from build123d import *

# Parameters (mm, degrees)
SKETCH2_R           = 6
BOSS_EXTRUDE1_DEPTH = 20


with BuildPart() as part:
    # Sketch2 → Boss-Extrude1 (new body)
    with BuildSketch(Plane(origin=(0, 0, 0), x_dir=(1, 0, 0), z_dir=(0, 1, 0))):
        with BuildLine():
            ThreePointArc((150, 0), (105, 77.942286341), (15, 77.942286341))
            ThreePointArc((15, 77.942286341), (7.764571353, 74.945273665), (0, 73.923048454))
            ThreePointArc((0, 73.923048454), (-7.764571353, 74.945273665), (-15, 77.942286341))
            ThreePointArc((-15, 77.942286341), (-150, 0), (-15, -77.942286341))
            ThreePointArc((-15, -77.942286341), (-7.764571353, -74.945273665), (0, -73.923048454))
            ThreePointArc((0, -73.923048454), (7.764571353, -74.945273665), (15, -77.942286341))
            ThreePointArc((15, -77.942286341), (105, -77.942286341), (150, 0))
        make_face()
        with Locations((60, 0)):
            Circle(SKETCH2_R, mode=Mode.SUBTRACT)
        with Locations((-60, 0)):
            Circle(SKETCH2_R, mode=Mode.SUBTRACT)
        with BuildLine():
            Line((5, 60.048226517), (5, 20))
            ThreePointArc((5, 20), (6.464466094, 16.464466094), (10, 15))
            Line((10, 15), (65.857864376, 15))
            ThreePointArc((65.857864376, 15), (67.771281538, 15.380602337), (69.393398282, 16.464466094))
            Line((69.393398282, 16.464466094), (109.023956198, 56.09502401))
            ThreePointArc((109.023956198, 56.09502401), (110.47724887, 59.964637812), (108.520983778, 63.605928444))
            ThreePointArc((108.520983778, 63.605928444), (65.119211843, 79.836042425), (20, 69.282032303))
            ThreePointArc((20, 69.282032303), (14.607936726, 66.68586026), (8.888888889, 64.923206732))
            ThreePointArc((8.888888889, 64.923206732), (6.0913202, 63.166274339), (5, 60.048226517))
        make_face(mode=Mode.SUBTRACT)
        with BuildLine():
            Line((134.330343737, 5), (73.036753237, 5))
            ThreePointArc((73.036753237, 5), (72.667201424, 5.246926627), (72.753910524, 5.682842712))
            Line((72.753910524, 5.682842712), (116.09502401, 49.023956198))
            ThreePointArc((116.09502401, 49.023956198), (119.964637812, 50.47724887), (123.605928444, 48.520983778))
            ThreePointArc((123.605928444, 48.520983778), (133.910362601, 30.614674589), (139.285699986, 10.666666667))
            ThreePointArc((139.285699986, 10.666666667), (138.094207, 6.708597057), (134.330343737, 5))
        make_face(mode=Mode.SUBTRACT)
        with BuildLine():
            Line((-72.753910524, 5.682842712), (-116.09502401, 49.023956198))
            ThreePointArc((-116.09502401, 49.023956198), (-119.964637812, 50.47724887), (-123.605928444, 48.520983778))
            ThreePointArc((-123.605928444, 48.520983778), (-133.910362601, 30.614674589), (-139.285699986, 10.666666667))
            ThreePointArc((-139.285699986, 10.666666667), (-138.094207, 6.708597057), (-134.330343737, 5))
            Line((-134.330343737, 5), (-73.036753237, 5))
            ThreePointArc((-73.036753237, 5), (-72.667201424, 5.246926627), (-72.753910524, 5.682842712))
        make_face(mode=Mode.SUBTRACT)
        with BuildLine():
            Line((-69.393398282, 16.464466094), (-109.023956198, 56.09502401))
            ThreePointArc((-109.023956198, 56.09502401), (-110.47724887, 59.964637812), (-108.520983778, 63.605928444))
            ThreePointArc((-108.520983778, 63.605928444), (-65.119211843, 79.836042425), (-20, 69.282032303))
            ThreePointArc((-20, 69.282032303), (-14.607936726, 66.68586026), (-8.888888889, 64.923206732))
            ThreePointArc((-8.888888889, 64.923206732), (-6.0913202, 63.166274339), (-5, 60.048226517))
            Line((-5, 60.048226517), (-5, 20))
            ThreePointArc((-5, 20), (-6.464466094, 16.464466094), (-10, 15))
            Line((-10, 15), (-65.857864376, 15))
            ThreePointArc((-65.857864376, 15), (-67.771281538, 15.380602337), (-69.393398282, 16.464466094))
        make_face(mode=Mode.SUBTRACT)
        with BuildLine():
            Line((-5, -60.048226517), (-5, -20))
            ThreePointArc((-5, -20), (-6.464466094, -16.464466094), (-10, -15))
            Line((-10, -15), (-65.857864376, -15))
            ThreePointArc((-65.857864376, -15), (-67.771281538, -15.380602337), (-69.393398282, -16.464466094))
            Line((-69.393398282, -16.464466094), (-109.023956198, -56.09502401))
            ThreePointArc((-109.023956198, -56.09502401), (-110.47724887, -59.964637812), (-108.520983778, -63.605928444))
            ThreePointArc((-108.520983778, -63.605928444), (-65.119211843, -79.836042425), (-20, -69.282032303))
            ThreePointArc((-20, -69.282032303), (-14.607936726, -66.68586026), (-8.888888889, -64.923206732))
            ThreePointArc((-8.888888889, -64.923206732), (-6.0913202, -63.166274339), (-5, -60.048226517))
        make_face(mode=Mode.SUBTRACT)
        with BuildLine():
            Line((-134.330343737, -5), (-73.036753237, -5))
            ThreePointArc((-73.036753237, -5), (-72.667201424, -5.246926627), (-72.753910524, -5.682842712))
            Line((-72.753910524, -5.682842712), (-116.09502401, -49.023956198))
            ThreePointArc((-116.09502401, -49.023956198), (-119.964637812, -50.47724887), (-123.605928444, -48.520983778))
            ThreePointArc((-123.605928444, -48.520983778), (-133.910362601, -30.614674589), (-139.285699986, -10.666666667))
            ThreePointArc((-139.285699986, -10.666666667), (-138.094207, -6.708597057), (-134.330343737, -5))
        make_face(mode=Mode.SUBTRACT)
        with BuildLine():
            Line((72.753910524, -5.682842712), (116.09502401, -49.023956198))
            ThreePointArc((116.09502401, -49.023956198), (119.964637812, -50.47724887), (123.605928444, -48.520983778))
            ThreePointArc((123.605928444, -48.520983778), (133.910362601, -30.614674589), (139.285699986, -10.666666667))
            ThreePointArc((139.285699986, -10.666666667), (138.094207, -6.708597057), (134.330343737, -5))
            Line((134.330343737, -5), (73.036753237, -5))
            ThreePointArc((73.036753237, -5), (72.667201424, -5.246926627), (72.753910524, -5.682842712))
        make_face(mode=Mode.SUBTRACT)
        with BuildLine():
            Line((69.393398282, -16.464466094), (109.023956198, -56.09502401))
            ThreePointArc((109.023956198, -56.09502401), (110.47724887, -59.964637812), (108.520983778, -63.605928444))
            ThreePointArc((108.520983778, -63.605928444), (65.119211843, -79.836042425), (20, -69.282032303))
            ThreePointArc((20, -69.282032303), (14.607936726, -66.68586026), (8.888888889, -64.923206732))
            ThreePointArc((8.888888889, -64.923206732), (6.0913202, -63.166274339), (5, -60.048226517))
            Line((5, -60.048226517), (5, -20))
            ThreePointArc((5, -20), (6.464466094, -16.464466094), (10, -15))
            Line((10, -15), (65.857864376, -15))
            ThreePointArc((65.857864376, -15), (67.771281538, -15.380602337), (69.393398282, -16.464466094))
        make_face(mode=Mode.SUBTRACT)
    extrude(amount=BOSS_EXTRUDE1_DEPTH)


solid = part.part
For this review, take the finished solid that the model builds, in its own axes (mm). Coordinates: 2 decimals unless noted, no trailing zeros. Loops run counter-clockwise (first coordinate to the right, second up) from the corner with the lowest first, then second, coordinate; pieces in that order, holes last. Notation, with made-up numbers: (58, 70) - (92, 70) arc R10 cw to (92, 78) - close; hole circle Ø5 at (-1, -28.5). An arc over 180 degrees is marked (long way). Use a Markdown table: item, result. Add a question column.
Item 1: Insertion check: pin 1 Ø12 at (y, z) = (12.5, 57.5) entering from +X; pin 2 Ø6 at (y, z) = (7, 50) entering from +X; pin 3 Ø6 at (x, y) = (-25.5, 14.5) entering from -Z; pin 4 Ø7 at (x, z) = (60, 0) entering from +Y. Each pin has a flat end and moves straight along its axis. Give the tip position at first contact, or say it passes through.
Item 2: We need section D-D (y = 9.75). Give the number of separate pieces and of enclosed holes in the cut face, and give its area (3 significant figures).
Item 3: We need section B-B (x = 60). Give the boundary of the cut face in (y, z).
Item 4: We need section A-A (z = 41.5). Give the boundary of the cut face in (x, y), and give its area (3 significant figures).
Item 5: For line 1 (X direction, y = 11, z = 0); line 2 (Z direction, x = 60, y = 7.75); line 3 (X direction, y = 7.25, z = 22.5), list the stretches that pass through material, from the lowest coordinate up.
Item 6: We need section C-C (x = -82.5). Give the boundary of the cut face in (y, z).
Results list:
| question | item | result |
|---|---|---|
| 1 | pin 1 | stops at x = 133.81 |
| 1 | pin 2 | stops at x = 136.75 |
| 1 | pin 3 | stops at z = -84.31 |
| 1 | pin 4 | passes through |
| 2 | separate pieces | 1 |
| 2 | enclosed holes | 10 |
| 2 | area | 17,000 mm^2 |
| 3 | outline | (0, -90) - (20, -90) - (20, -80) - (0, -80) - close; (0, -15) - (20, -15) - (20, -6) - (0, -6) - close; (0, 6) - (20, 6) - (20, 15) - (0, 15) - close; (0, 80) - (20, 80) - (20, 90) - (0, 90) - close |
| 4 | outline | (-139.86, 0) - (-128.39, 0) - (-128.39, 20) - (-139.86, 20) - close; (-108.57, 0) - (-94.43, 0) - (-94.43, 20) - (-108.57, 20) - close; (-5, 0) - (5, 0) - (5, 20) - (-5, 20) - close; (94.43, 0) - (108.57, 0) - (108.57, 20) - (94.43, 20) - close; (128.39, 0) - (139.86, 0) - (139.86, 20) - (128.39, 20) - close |
| 4 | area | 1,220 mm^2 |
| 5 | line 1 | x = -150 to -66, -54 to 54, 66 to 150 |
| 5 | line 2 | z = -90 to -80, -15 to -6, 6 to 15, 80 to 90 |
| 5 | line 3 | x = -147.14 to -136.77, -89.57 to -75.43, -5 to 5, 75.43 to 89.57, 136.77 to 147.14 |
| 6 | outline | (0, -87.14) - (20, -87.14) - (20, -76.77) - (0, -76.77) - close; (0, -29.57) - (20, -29.57) - (20, -15.43) - (0, -15.43) - close; (0, -5) - (20, -5) - (20, 5) - (0, 5) - close; (0, 15.43) - (20, 15.43) - (20, 29.57) - (0, 29.57) - close; (0, 76.77) - (20, 76.77) - (20, 87.14) - (0, 87.14) - close |
